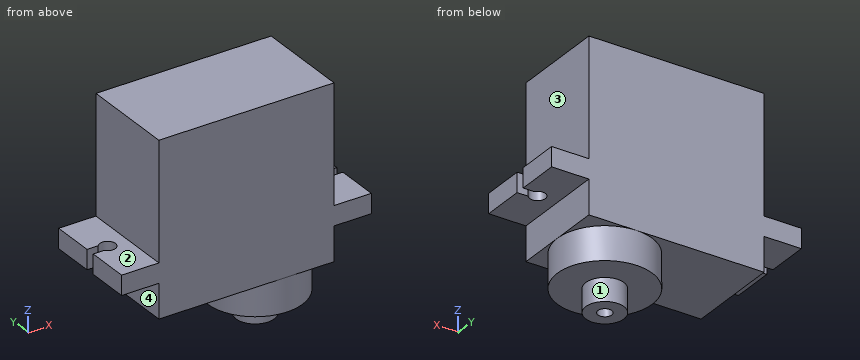
```python
from build123d import *

# Parameters (mm, degrees)
SKETCH1_W           = 22.8
SKETCH1_H           = 22.3
BOSS_EXTRUDE1_DEPTH = 6.175
SKETCH2_W           = 2.54
SKETCH2_H           = 12.35
BOSS_EXTRUDE2_DEPTH = 4.85
CUT_EXTRUDE1_DEPTH  = 18.84
SKETCH4_R           = 6.175
BOSS_EXTRUDE3_DEPTH = 4.35
SKETCH5_R           = 2.475
BOSS_EXTRUDE4_DEPTH = 3
SKETCH6_R           = 0.9
CUT_EXTRUDE2_DEPTH  = 2


with BuildPart() as part:
    # Sketch1 → Boss-Extrude1 (new body, symmetric)
    with BuildSketch(Plane(origin=(0, 0, 0), x_dir=(1, 0, 0), z_dir=(0, 1, 0))):
        Rectangle(SKETCH1_W, SKETCH1_H)
    extrude(amount=BOSS_EXTRUDE1_DEPTH, both=True)

    # Sketch2 → Boss-Extrude2 (add)
    with BuildSketch(Plane(origin=(11.4, 0, 0), x_dir=(0, 0, -1), z_dir=(1, 0, 0))):
        with Locations((5.42, 0)):
            Rectangle(SKETCH2_W, SKETCH2_H)
    boss_extrude2 = extrude(amount=BOSS_EXTRUDE2_DEPTH)

    # Mirror1: Boss-Extrude2 across plane
    add(boss_extrude2.mirror(Plane(origin=(0, 0, 0), x_dir=(0, 0, 1), z_dir=(1, 0, 0))))

    # Sketch3 → Cut-Extrude1 (cut, through all)
    with BuildSketch(Plane(origin=(0, 0, -6.69), x_dir=(-1, 0, 0), z_dir=(0, 0, -1))):
        with BuildLine():
            Line((-14.806038507, 0.6), (-16.25, 0.6))
            Line((-16.25, 0.6), (-16.25, -0.6))
            Line((-16.25, -0.6), (-14.806038507, -0.6))
            ThreePointArc((-14.806038507, -0.6), (-12.95, 0), (-14.806038507, 0.6))
        make_face()
        with BuildLine():
            Line((14.806038507, 0.6), (16.25, 0.6))
            Line((16.25, 0.6), (16.25, -0.6))
            Line((16.25, -0.6), (14.806038507, -0.6))
            ThreePointArc((14.806038507, -0.6), (12.95, 0), (14.806038507, 0.6))
        make_face()
    extrude(amount=-CUT_EXTRUDE1_DEPTH, mode=Mode.SUBTRACT)

    # Sketch4 → Boss-Extrude3 (add)
    with BuildSketch(Plane(origin=(0, 0, -11.15), x_dir=(-1, 0, 0), z_dir=(0, 0, -1))):
        with Locations((-5.225, 0)):
            Circle(SKETCH4_R)
    extrude(amount=BOSS_EXTRUDE3_DEPTH)

    # Sketch5 → Boss-Extrude4 (add)
    with BuildSketch(Plane(origin=(0, 0, -15.5), x_dir=(-1, 0, 0), z_dir=(0, 0, -1))):
        with Locations((-5.225, 0)):
            Circle(SKETCH5_R)
    extrude(amount=BOSS_EXTRUDE4_DEPTH)

    # Sketch6 → Cut-Extrude2 (cut)
    with BuildSketch(Plane(origin=(0, 0, -18.5), x_dir=(-1, 0, 0), z_dir=(0, 0, -1))):
        with Locations((-5.225, 0)):
            Circle(SKETCH6_R)
    extrude(amount=-CUT_EXTRUDE2_DEPTH, mode=Mode.SUBTRACT)


solid = part.part
```
Here's how the part is built. I have some questions about the finished solid (model axes, mm). Face numbers are marked on the shaded views. A direction names the side the tool comes from. Coordinates: 2 decimals unless noted, no trailing zeros. Order: outer loops, then holes, each group sorted by start corner. A loop starts at its lowest first (then second) coordinate and runs counter-clockwise, first axis right, second up.
1) Which directions (+Z, -Z, +X, -X, +Y, -Y) give clear straight access to the entire face, cutting with the end or side of a thin tool? Please do the marked faces 1, 2, 3 and 4.
2) Imagine slicing it at C-C on z = -2.25. List the corners of the cut face in (x, y) for me (3 decimals).
3) Imagine slicing it at B-B on x = 0. List the corners of the cut face in (y, z) for me (3 decimals).
4) Imagine slicing it at A-A on y = 3. List the corners of the cut face in (x, z) for me, and give its area (3 significant figures).
5) Will these pins go through, and if not, where does the flat tip stop? pin 1 (1.9 mm diameter, centred on x = 7, y = -2, fed in from -Z); pin 2 (3 mm diameter, centred on y = -4.5, z = -12.5, fed in from +X); pin 3 (2.5 mm diameter, centred on x = -13.975, y = 0, fed in from -Z); pin 4 (1.5 mm diameter, centred on x = -14.5, y = 2, fed in from +Z).
6) I need wall thicknesses on line 1 (Z direction, x = -7, y = 3.25); line 2 (Z direction, x = -11.5, y = 1.5); line 3 (Y direction, x = -15, z = -5.75) (3 decimals). Which ranges of each line are inside material? Lowest first, please.
7) Imagine slicing it at D-D on y = -4. List the corners of the cut face in (x, z) for me.
Response values:
1. face 1: -Z
1. face 2: +Z, -X, +Y, -Y
1. face 3: +Z, +X, +Y, -Y
1. face 4: -Z, -X, +Y, -Y
2. outline: (-11.4, -6.175) - (11.4, -6.175) - (11.4, 6.175) - (-11.4, 6.175) - close
3. outline: (-6.175, -11.15) - (-3.291, -11.15) - (-3.291, -15.5) - (3.291, -15.5) - (3.291, -11.15) - (6.175, -11.15) - (6.175, 11.15) - (-6.175, 11.15) - close
4. outline: (-16.25, -6.69) - (-11.4, -6.69) - (-11.4, -11.15) - (-0.17, -11.15) - (-0.17, -15.5) - (10.62, -15.5) - (10.62, -11.15) - (11.4, -11.15) - (11.4, -6.69) - (16.25, -6.69) - (16.25, -4.15) - (11.4, -4.15) - (11.4, 11.15) - (-11.4, 11.15) - (-11.4, -4.15) - (-16.25, -4.15) - close
4. area: 580 mm2
5. pin 1: stops at z = -18.5
5. pin 2: stops at x = 11.4
5. pin 3: stops at z = -6.69
5. pin 4: stops at z = -4.15
6. line 1: z = -11.15 to 11.15
6. line 2: z = -6.69 to -4.15
6. line 3: y = -6.175 to -0.6, 0.6 to 6.175
7. outline: (-16.25, -6.69) - (-11.4, -6.69) - (-11.4, -11.15) - (0.52, -11.15) - (0.52, -15.5) - (9.93, -15.5) - (9.93, -11.15) - (11.4, -11.15) - (11.4, -6.69) - (16.25, -6.69) - (16.25, -4.15) - (11.4, -4.15) - (11.4, 11.15) - (-11.4, 11.15) - (-11.4, -4.15) - (-16.25, -4.15) - close
